Design review of the part shown in the three views and the two pictorial views. Dimensions are in mm from the part's minimum x, y and z. A direction names the side the tool comes from. Round coordinates to 2 decimals unless told otherwise and drop trailing zeros. Loops run counter-clockwise (first coordinate to the right, second up) from the corner with the lowest first, then second, coordinate; pieces in that order, holes last. Notation, with made-up numbers: (80.25, -9) -> (118.25, -9) arc R28 ccw to (118.25, 11) -> close; hole circle Ø10 at (19.25, -0.5). An arc over 180 degrees is marked (long way). Use a Markdown table: item, result. Add a question column.
1) For the marked faces 4, 5 and 6, list the 3-axis set-ups (+Z, -Z, +X, -X, +Y, -Y) from which the entire face can be reached by the end or side of a thin tool; tool diameter is ignored.
2) Consider section D-D on z = 20. Give the boundary of the cut face in (x, y), plus the area to 3 significant figures.
3) Consider section A-A on x = 17. Give the boundary of the cut face in (y, z), plus the area to 3 significant figures.
4) Wall thickness on probe 1 along Z at (x, y) = (9.5, 2.5); probe 2 along Y at (x, z) = (43.5, 20.5); probe 3 along Y at (x, z) = (18, 3): over which ranges is each line inside the solid? List them lowest first.
5) Insertion check: pin 1 (1 mm diameter, centred on y = 6.5, z = 41, fed in from +X); pin 2 (2 mm diameter, centred on y = 10, z = 54, fed in from -X); pin 3 (8 mm diameter, centred on x = 17.5, y = 9.5, fed in from -Z); pin 4 (12 mm diameter, centred on x = 30.5, z = 51, fed in from +Y). Each pin has a flat end and moves straight along its axis. Give the tip position at first contact, or say it passes through.
6) Mouldability with a two-part tool opening along Z and no side actions: class the marked faces 1, 2 and 3 as released by +Z, released by -Z, zero draft, split by the parting line, or undercut.
7) Consider section C-C on y = 1.5. Give the boundary of the cut face in (x, z), plus the area to 3 significant figures.
8) Consider section B-B on z = 33. Give the boundary of the cut face in (x, y) (1 decimal).
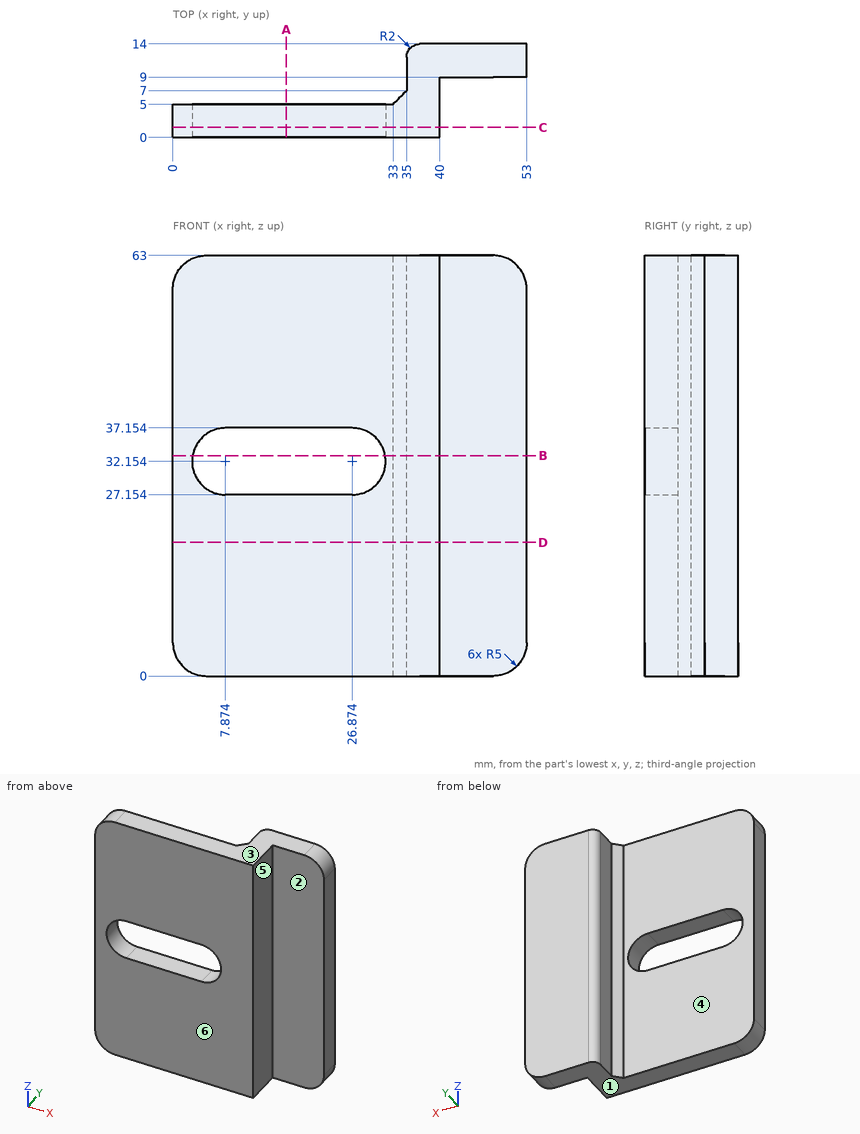
Result set:
| question | item | result |
|---|---|---|
| 1 | face 4 | +Z, -Z, -X, +Y |
| 1 | face 5 | +Z, -Z, +X, -Y |
| 1 | face 6 | +Z, -Z, +X, -X, -Y |
| 2 | outline | (0, 0) -> (40, 0) -> (40, 9) -> (53, 9) -> (53, 14) -> (37, 14) arc R2 ccw to (35, 12) -> (35, 7) -> (33, 5) -> (0, 5) -> close |
| 2 | area | 311 mm2 |
| 3 | outline | (0, 0) -> (5, 0) -> (5, 27.15) -> (0, 27.15) -> close; (0, 37.15) -> (5, 37.15) -> (5, 63) -> (0, 63) -> close |
| 3 | area | 265 mm2 |
| 4 | probe 1 | 0 to 27.15, 37.15 to 63 |
| 4 | probe 2 | 9 to 14 |
| 4 | probe 3 | 0 to 5 |
| 5 | pin 1 | x = 40 |
| 5 | pin 2 | x = 35 |
| 5 | pin 3 | through |
| 5 | pin 4 | y = 13.94 |
| 6 | face 1 | released by -Z |
| 6 | face 2 | zero draft |
| 6 | face 3 | released by +Z |
| 7 | outline | (0, 5) arc R5 ccw to (5, 0) -> (40, 0) -> (40, 63) -> (5, 63) arc R5 ccw to (0, 58) -> close; hole (7.87, 27.15) -> (26.87, 27.15) arc R5 ccw to (26.87, 37.15) -> (7.87, 37.15) arc R5 ccw to start |
| 7 | area | 2,240 mm2 |
| 8 | outline | (0, 0) -> (2.9, 0) -> (2.9, 5) -> (0, 5) -> close; (31.8, 0) -> (40, 0) -> (40, 9) -> (53, 9) -> (53, 14) -> (37, 14) arc R2 ccw to (35, 12) -> (35, 7) -> (33, 5) -> (31.8, 5) -> close |
